from build123d import *

# Parameters (mm, degrees)
BOSS_EXTRUDE1_DEPTH  = 38.1
HOLE1_D              = 9.525
HOLE1_DEPTH          = 101.6
HOLE2_D              = 3.175
HOLE2_DEPTH          = 101.6
LPATTERN1_COUNT      = 2
LPATTERN1_PITCH      = 20.32
LPATTERN1_COUNT_DIR2 = 2
LPATTERN1_PITCH_DIR2 = 114.3


with BuildPart() as part:
    # Sketch1 → Boss-Extrude1 (new body)
    with BuildSketch(Plane.XY):
        with BuildLine():
            Line((-63.5, 0), (63.5, 0))
            Line((63.5, 0), (63.5, 15.24))
            Line((63.5, 15.24), (49.53, 15.24))
            ThreePointArc((49.53, 15.24), (48.224317592, 9.934993562), (44.605574225, 5.842))
            Line((44.605574225, 5.842), (31.594425775, 5.842))
            ThreePointArc((31.594425775, 5.842), (27.975682408, 9.934993562), (26.67, 15.24))
            Line((26.67, 15.24), (-26.67, 15.24))
            ThreePointArc((-26.67, 15.24), (-27.975682408, 9.934993562), (-31.594425775, 5.842))
            Line((-31.594425775, 5.842), (-44.605574225, 5.842))
            ThreePointArc((-44.605574225, 5.842), (-48.224317592, 9.934993562), (-49.53, 15.24))
            Line((-49.53, 15.24), (-63.5, 15.24))
            Line((-63.5, 15.24), (-63.5, 0))
        make_face()
    extrude(amount=BOSS_EXTRUDE1_DEPTH)

    # Hole1
    with Locations(Plane(origin=(0, 15.24, 0), x_dir=(1, 0, 0), z_dir=(0, 1, 0))):
        with Locations((0, -19.05)):
            Hole(HOLE1_D / 2, depth=HOLE1_DEPTH)

    # Hole2
    with Locations(Plane(origin=(0, 15.24, 0), x_dir=(1, 0, 0), z_dir=(0, 1, 0))):
        with Locations((-57.15, -8.89)):
            hole2 = Hole(HOLE2_D / 2, depth=HOLE2_DEPTH)

    # LPattern1: Hole2 2 × 2
    with Locations(*[(j * LPATTERN1_PITCH_DIR2, 0, i * LPATTERN1_PITCH) for i in range(LPATTERN1_COUNT) for j in range(LPATTERN1_COUNT_DIR2) if (i, j) != (0, 0)]):
        add(hole2, mode=Mode.SUBTRACT)


solid = part.part
Geometry: final body of the model. Coordinates: model frame, mm. A direction names the side the tool comes from. Coordinates: 2 decimals unless noted, no trailing zeros. Order: outer loops, then holes, each group sorted by start corner. A loop starts at its lowest first (then second) coordinate and runs counter-clockwise, first axis right, second up. Notation, with made-up numbers: M 88,61.25 L 140,61.25 A11 ccw 140,70.25 Z; hole C 55.25,62 d7. An arc over 180 degrees is marked long. One line per question, with ' | ' between items. Start each with the question number.
Item 1: Cut plane D-D, the plane z = 8.89. Return the cut outline in (x, y).
Item 2: Ray query, probe 1 along Z at (x, y) = (-57.15, 10.5); probe 2 along X at (y, z) = (3.75, 29); probe 3 along X at (y, z) = (8, 19). Return the intervals inside material, ascending. Write a range as [from, to].
Item 3: Cut plane A-A, the plane x = 0. Return the cut outline in (y, z).
Item 4: Draft query along Z for faces 1 (the cylindrical face through (-58.664, 7.513, 8.413)), 2 (the flat face through (-38, 5.842, 19)), 3 (the flat face through (-1, 6, 38.1)). Return one class per face: released by +Z, released by -Z, zero draft, split by the parting line, or undercut.
Item 5: Cut plane C-C, the plane x = 57.15. Return the cut outline in (y, z), then the cut area to 3 significant figures.
Item 6: Set-up query: faces 4 (the flat face through (38, 5.842, 19)), 5 (the flat face through (-63.5, 8, 19)). Return all of +Z, -Z, +X, -X, +Y, -Y with unobstructed straight access to the full face (end or side cutting, diameter ignored); none if empty.
Item 7: Cut plane B-B, the plane y = 10.5. Count the separate pieces of the cut face and the enclosed holes in it, then the cut area to 3 significant figures.
Item 8: Pin query (flat end, axial travel): pin 1 Ø5 at (x, y) = (42.5, 6) entering from -Z; pin 2 Ø6.5 at (x, z) = (40, 13.5) entering from +Y. Return the tip coordinate at first contact, or that it passes through.
A:
1) outline: M -63.5,0 L -58.74,0 L -58.74,15.24 L -63.5,15.24 Z; M -55.56,0 L 55.56,0 L 55.56,15.24 L 49.53,15.24 A11.43 cw 44.61,5.84 L 31.59,5.84 A11.43 cw 26.67,15.24 L -26.67,15.24 A11.43 cw -31.59,5.84 L -44.61,5.84 A11.43 cw -49.53,15.24 L -55.56,15.24 Z; M 58.74,0 L 63.5,0 L 63.5,15.24 L 58.74,15.24 Z
2) probe 1: z = [0, 7.3], [10.48, 27.62], [30.8, 38.1] | probe 2: x = [-63.5, -58.72], [-55.58, 55.58], [58.72, 63.5] | probe 3: x = [-63.5, -46.94], [-29.26, -4.76], [4.76, 29.26], [46.94, 63.5]
3) outline: M 0,0 L 15.24,0 L 15.24,14.29 L 0,14.29 Z; M 0,23.81 L 15.24,23.81 L 15.24,38.1 L 0,38.1 Z
4) face 1: undercut | face 2: zero draft | face 3: released by +Z
5) outline: M 0,0 L 15.24,0 L 15.24,7.3 L 0,7.3 Z; M 0,10.48 L 15.24,10.48 L 15.24,27.62 L 0,27.62 Z; M 0,30.8 L 15.24,30.8 L 15.24,38.1 L 0,38.1 Z | area: 484 mm2
6) face 4: +Z, -Z, +Y | face 5: +Z, -Z, -X, +Y, -Y
7) separate pieces: 3 | enclosed holes: 5 | area: 3,150 mm2
8) pin 1: stops at z = 0 | pin 2: stops at y = 5.84
